```python
from build123d import *

# Parameters (mm, degrees)
F0_W          = 30
F0_H          = 30
F0_W_2        = 24
F0_H_2        = 24
F1_DEPTH      = 30
F3_DEPTH      = 5
F5_DEPTH      = 4
F6_W          = 12
F6_H          = 5
F6_W_2        = 6
F6_W_3        = 3
F6_W_4        = 24
F7_DEPTH      = 3
F8_W          = 30.8
F8_H          = 30.8
F8_W_2        = 27
F8_H_2        = 27
F9_DEPTH      = 1
F10_T1_DEPTH  = 27
F10_T3_DEPTH  = 27
F10_T9_DEPTH  = 30.7080992435
F10_T14_DEPTH = 30.7080992435
F10_T22_DEPTH = 30.7080992435
F10_T27_DEPTH = 30.7080992435
F10_T35_DEPTH = 30.7080992435
F10_T40_DEPTH = 30.7080992435
F10_T48_DEPTH = 30.7080992435
F10_T53_DEPTH = 30.7080992435
F11_T1_DEPTH  = 55


# Not quite as in the source:
# - a fillet or chamfer that OpenCascade refuses, or shapes differently, is made with other operations: its cross-section is extruded or revolved along the edge and cut away or added


with BuildPart() as f1:
    # F0 (on Top) → F1 (new body)
    with BuildSketch(Plane.XY):
        Rectangle(F0_W, F0_H)
        Rectangle(F0_W_2, F0_H_2, mode=Mode.SUBTRACT)
    extrude(amount=F1_DEPTH)

    # F2 (on face) → F3 (cut)
    with BuildSketch(Plane.XZ.offset(15)):
        Polygon((11, 22.7017059222), (-11, 10), (11, 10), align=None)
    extrude(amount=-F3_DEPTH, mode=Mode.SUBTRACT)

    # F4 (on face) → F5 (cut)
    with BuildSketch(Plane(origin=(-15, 0, 0), x_dir=(0, -1, 0), z_dir=(-1, 0, 0))):
        with BuildLine():
            ThreePointArc((11, 2), (6.0293863659, 20.1017884635), (-11, 28))
            Line((-11, 28), (-11, 2))
            Line((-11, 2), (11, 2))
        make_face()
    extrude(amount=-F5_DEPTH, mode=Mode.SUBTRACT)

    # F6 (on face) → F7 (cut)
    with BuildSketch(Plane(origin=(0, 15, 0), x_dir=(-1, 0, 0), z_dir=(0, 1, 0))):
        with Locations((6, 18.5)):
            Rectangle(F6_W, F6_H)
        with Locations((9, 11.5)):
            Rectangle(F6_W_2, F6_H)
        with Locations((10.5, 4.5)):
            Rectangle(F6_W_3, F6_H)
        with Locations((0, 25.5)):
            Rectangle(F6_W_4, F6_H)
    extrude(amount=-F7_DEPTH, mode=Mode.SUBTRACT)

    # F8 (on face) → F9 (cut)
    with BuildSketch(Plane(origin=(0, 0, 0), x_dir=(1, 0, 0), z_dir=(0, 0, -1))):
        Rectangle(F8_W, F8_H)
        Rectangle(F8_W_2, F8_H_2, mode=Mode.SUBTRACT)
    extrude(amount=-F9_DEPTH, mode=Mode.SUBTRACT)

    # F10: fillet of radius 1.6 on 4 edges, made by hand

    # F10_s2 → F10_t1 (join)
    with BuildSketch(Plane.XZ.offset(-13.5)):
        with BuildLine():
            ThreePointArc((-14.9832396974, 1), (-14.0888125064, 0.7266499161), (-13.5, 0))
            Line((-13.5, 0), (-13.5, 1))
            Line((-13.5, 1), (-14.9832396974, 1))
        make_face()
        with BuildLine():
            ThreePointArc((14.9832396974, 1), (14.0888125064, 0.7266499161), (13.5, 0))
            Line((13.5, 0), (13.5, 1))
            Line((13.5, 1), (14.9832396974, 1))
        make_face()
    extrude(amount=F10_T1_DEPTH)

    # F10_s4 → F10_t3 (join)
    with BuildSketch(Plane.YZ.offset(-13.5)):
        with BuildLine():
            ThreePointArc((14.9832396974, 1), (14.0888125064, 0.7266499161), (13.5, 0))
            Line((13.5, 0), (13.5, 1))
            Line((13.5, 1), (14.9832396974, 1))
        make_face()
        with BuildLine():
            ThreePointArc((-14.9832396974, 1), (-14.0888125064, 0.7266499161), (-13.5, 0))
            Line((-13.5, 0), (-13.5, 1))
            Line((-13.5, 1), (-14.9832396974, 1))
        make_face()
    extrude(amount=F10_T3_DEPTH)


with BuildPart() as f10_tool7:
    # F10_s8 → F10_t9 (new body)
    with BuildSketch(Plane.XZ.offset(-17.2080992435)):
        with BuildLine():
            ThreePointArc((-14.9832396974, 1), (-14.0888125064, 0.7266499161), (-13.5, 0))
            Line((-13.5, 0), (-13.5, 1))
            Line((-13.5, 1), (-14.9832396974, 1))
        make_face()
    extrude(amount=F10_T9_DEPTH)

    split(bisect_by=Plane.XZ.offset(-15), keep=Keep.TOP)

    split(bisect_by=Plane.XZ.offset(-13.5), keep=Keep.BOTTOM)


with BuildPart() as f10_tool12:
    # F10_s13 → F10_t14 (new body)
    with BuildSketch(Plane.YZ.offset(13.5)):
        with BuildLine():
            ThreePointArc((14.9832396974, 1), (14.0888125064, 0.7266499161), (13.5, 0))
            Line((13.5, 0), (13.5, 1))
            Line((13.5, 1), (14.9832396974, 1))
        make_face()
    extrude(amount=-F10_T14_DEPTH)

    split(bisect_by=Plane.YZ.offset(-15), keep=Keep.TOP)

    split(bisect_by=Plane.YZ.offset(-13.5), keep=Keep.BOTTOM)


with BuildPart() as f10_tool7_1:
    add(f10_tool7.part)

    # F10_t17: intersect F10_tool12
    add(f10_tool12.part, mode=Mode.INTERSECT)


with BuildPart() as f1_1:
    add(f1.part)

    # F10_t5: union F10_tool7
    add(f10_tool7_1.part)


with BuildPart() as f10_tool20:
    # F10_s21 → F10_t22 (new body)
    with BuildSketch(Plane.XZ.offset(-13.5)):
        with BuildLine():
            ThreePointArc((-14.9832396974, 1), (-14.0888125064, 0.7266499161), (-13.5, 0))
            Line((-13.5, 0), (-13.5, 1))
            Line((-13.5, 1), (-14.9832396974, 1))
        make_face()
    extrude(amount=F10_T22_DEPTH)

    split(bisect_by=Plane.XZ.offset(15), keep=Keep.BOTTOM)

    split(bisect_by=Plane.XZ.offset(13.5), keep=Keep.TOP)


with BuildPart() as f10_tool25:
    # F10_s26 → F10_t27 (new body)
    with BuildSketch(Plane.YZ.offset(-17.2080992435)):
        with BuildLine():
            ThreePointArc((-14.9832396974, 1), (-14.0888125064, 0.7266499161), (-13.5, 0))
            Line((-13.5, 0), (-13.5, 1))
            Line((-13.5, 1), (-14.9832396974, 1))
        make_face()
    extrude(amount=F10_T27_DEPTH)

    split(bisect_by=Plane.YZ.offset(-15), keep=Keep.TOP)

    split(bisect_by=Plane.YZ.offset(-13.5), keep=Keep.BOTTOM)


with BuildPart() as f10_tool20_1:
    add(f10_tool20.part)

    # F10_t30: intersect F10_tool25
    add(f10_tool25.part, mode=Mode.INTERSECT)


with BuildPart() as f1_2:
    add(f1_1.part)

    # F10_t18: union F10_tool20
    add(f10_tool20_1.part)


with BuildPart() as f10_tool33:
    # F10_s34 → F10_t35 (new body)
    with BuildSketch(Plane.YZ.offset(17.2080992435)):
        with BuildLine():
            ThreePointArc((14.9832396974, 1), (14.0888125064, 0.7266499161), (13.5, 0))
            Line((13.5, 0), (13.5, 1))
            Line((13.5, 1), (14.9832396974, 1))
        make_face()
    extrude(amount=-F10_T35_DEPTH)

    split(bisect_by=Plane.YZ.offset(15), keep=Keep.BOTTOM)

    split(bisect_by=Plane.YZ.offset(13.5), keep=Keep.TOP)


with BuildPart() as f10_tool38:
    # F10_s39 → F10_t40 (new body)
    with BuildSketch(Plane.XZ.offset(13.5)):
        with BuildLine():
            ThreePointArc((14.9832396974, 1), (14.0888125064, 0.7266499161), (13.5, 0))
            Line((13.5, 0), (13.5, 1))
            Line((13.5, 1), (14.9832396974, 1))
        make_face()
    extrude(amount=-F10_T40_DEPTH)

    split(bisect_by=Plane.XZ.offset(-15), keep=Keep.TOP)

    split(bisect_by=Plane.XZ.offset(-13.5), keep=Keep.BOTTOM)


with BuildPart() as f10_tool33_1:
    add(f10_tool33.part)

    # F10_t43: intersect F10_tool38
    add(f10_tool38.part, mode=Mode.INTERSECT)


with BuildPart() as f1_3:
    add(f1_2.part)

    # F10_t31: union F10_tool33
    add(f10_tool33_1.part)


with BuildPart() as f10_tool46:
    # F10_s47 → F10_t48 (new body)
    with BuildSketch(Plane.YZ.offset(-13.5)):
        with BuildLine():
            ThreePointArc((-14.9832396974, 1), (-14.0888125064, 0.7266499161), (-13.5, 0))
            Line((-13.5, 0), (-13.5, 1))
            Line((-13.5, 1), (-14.9832396974, 1))
        make_face()
    extrude(amount=F10_T48_DEPTH)

    split(bisect_by=Plane.YZ.offset(15), keep=Keep.BOTTOM)

    split(bisect_by=Plane.YZ.offset(13.5), keep=Keep.TOP)


with BuildPart() as f10_tool51:
    # F10_s52 → F10_t53 (new body)
    with BuildSketch(Plane.XZ.offset(17.2080992435)):
        with BuildLine():
            ThreePointArc((14.9832396974, 1), (14.0888125064, 0.7266499161), (13.5, 0))
            Line((13.5, 0), (13.5, 1))
            Line((13.5, 1), (14.9832396974, 1))
        make_face()
    extrude(amount=-F10_T53_DEPTH)

    split(bisect_by=Plane.XZ.offset(15), keep=Keep.BOTTOM)

    split(bisect_by=Plane.XZ.offset(13.5), keep=Keep.TOP)


with BuildPart() as f10_tool46_1:
    add(f10_tool46.part)

    # F10_t56: intersect F10_tool51
    add(f10_tool51.part, mode=Mode.INTERSECT)


with BuildPart() as f1_4:
    add(f1_3.part)

    # F10_t44: union F10_tool46
    add(f10_tool46_1.part)

    # F11: fillet of radius 5 on 1 edges, made by hand

    # F11_s2 → F11_t1 (cut)
    with BuildSketch(Plane.XZ.offset(-27.5)):
        with BuildLine():
            ThreePointArc((15, 25), (13.5355339059, 28.5355339059), (10, 30))
            Line((10, 30), (15, 30))
            Line((15, 30), (15, 25))
        make_face()
    extrude(amount=F11_T1_DEPTH, mode=Mode.SUBTRACT)


solid = f1_4.part
```
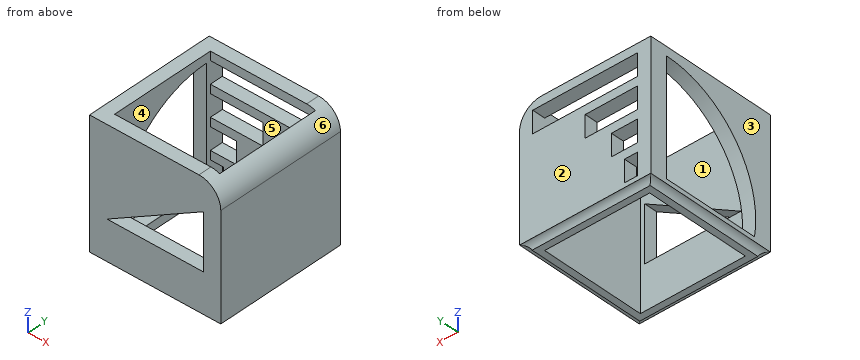
Input: part model. Units: mm. Frame: model coordinates. Face numbers are marked on the shaded views. A direction names the side the tool comes from. Give positions to 0.01 mm unless a question says otherwise; leave off trailing zeros. Order: outer loops, then holes, each group sorted by start corner. A loop starts at its lowest first (then second) coordinate and runs counter-clockwise, first axis right, second up.
1. Reachability of the marked faces 4, 5 and 6 from +Z, -Z, +X, -X, +Y, -Y: full face, straight path, thin tool, end or side. Return the list, or none.
Derived:
face 4: none
face 5: +Z, -Z
face 6: +Z, +X, +Y, -Y
2. Section B-B on z = 10.5. Return the cut outline in (x, y).
Derived:
outline: (-15, -15) - (-10.13, -15) - (-10.13, -12) - (-12, -12) - (-12, -10.78) - (-15, -10.78) - close; (-15, 11) - (-12, 11) - (-12, 15) - (-15, 15) - close; (-6, 12) - (12, 12) - (12, -12) - (11, -12) - (11, -15) - (15, -15) - (15, 15) - (-6, 15) - close
3. Material intervals for L1, parallel to Y at x = 0.75, z = 8; L2, parallel to Z at x = -0.5, y = 13.75, sorted ascending.
Derived:
L1: y = -15 to -12, 12 to 15
L2: z = 0.42 to 16, 21 to 23, 28 to 30
4. Section A-A on x = -9.5. Give the number of separate pieces and of enclosed holes in the cut face, and give its area (3 significant figures).
Derived:
separate pieces: 7
enclosed holes: 0
area: 115 mm2
5. Mould query, pull axis Y, two halves, no side actions, for the marked faces 1, 2 and 3. Classes: released by +Y, released by -Y, zero draft, split by the parting line, or undercut.
Derived:
face 1: undercut
face 2: released by +Y
face 3: zero draft
6. Pin query (flat end, axial travel): pin 1 (3 mm diameter, centred on y = 4, z = 19.5, fed in from -X); pin 2 (12 mm diameter, centred on x = 2, y = -3, fed in from -Z). Return the tip coordinate at first contact, or that it passes through.
Derived:
pin 1: stops at x = 12
pin 2: passes through
